from build123d import *

# Parameters (mm, degrees)
SKETCH1_W           = 203.2
SKETCH1_H           = 152.4
BOSS_EXTRUDE1_DEPTH = 12.7
SKETCH2_R           = 2.778125
CUT_EXTRUDE1_DEPTH  = 255.31730181
LPATTERN1_COUNT     = 4
LPATTERN1_PITCH     = 50.8
SKETCH4_R           = 2.778125
SKETCH4_R_2         = 3.175
CUT_EXTRUDE2_DEPTH  = 255.31730181


with BuildPart() as part:
    # Sketch1 → Boss-Extrude1 (new body)
    with BuildSketch(Plane(origin=(0, 0, 0), x_dir=(1, 0, 0), z_dir=(0, 1, 0))):
        with Locations((101.6, 76.2)):
            Rectangle(SKETCH1_W, SKETCH1_H)
    extrude(amount=BOSS_EXTRUDE1_DEPTH)

    # Sketch2 → Cut-Extrude1 (cut, through all)
    with BuildSketch(Plane(origin=(0, 12.7, 0), x_dir=(1, 0, 0), z_dir=(0, 1, 0))):
        with Locations(Location((25.4, 139.7, 0), (0, 0, 270))):
            Circle(SKETCH2_R)
        with Locations(Location((25.4, 12.7, 0), (0, 0, 270))):
            Circle(SKETCH2_R)
    cut_extrude1 = extrude(amount=-CUT_EXTRUDE1_DEPTH, mode=Mode.SUBTRACT)

    # LPattern1: Cut-Extrude1 ×4
    with Locations(*[(i * LPATTERN1_PITCH, 0, 0) for i in range(1, LPATTERN1_COUNT)]):
        add(cut_extrude1, mode=Mode.SUBTRACT)

    # Sketch4 → Cut-Extrude2 (cut, through all)
    with BuildSketch(Plane(origin=(0, 12.7, 0), x_dir=(1, 0, 0), z_dir=(0, 1, 0))):
        with Locations(Location((53.975, 76.2, 0), (0, 0, 270))):
            Circle(SKETCH4_R)
        with Locations(Location((53.34, 107.95, 0), (0, 0, 270))):
            Circle(SKETCH4_R)
        with Locations(Location((101.6, 50.8, 0), (0, 0, 270))):
            Circle(SKETCH4_R_2)
        with Locations(Location((142.875, 107.95, 0), (0, 0, 270))):
            Circle(SKETCH4_R)
        with Locations(Location((136.525, 53.975, 0), (0, 0, 270))):
            Circle(SKETCH4_R)
    extrude(amount=-CUT_EXTRUDE2_DEPTH, mode=Mode.SUBTRACT)


solid = part.part
Can you work these out from the model? Positions are in its coordinate system, mm. Coordinates: 2 decimals unless noted, no trailing zeros. Write each loop counter-clockwise with the first axis right and the second up, starting at its lowest first coordinate (ties: lowest second). Pieces come first, ordered by that corner, then holes. Notation, with made-up numbers: (-26, 68) -> (12, 68) arc R7 ccw to (12, 81) -> close; hole circle Ø3 at (-38.75, 10.25). An arc over 180 degrees is marked (long way). Write each question's results on one line, items separated by ' | '. Start each with the question number.
Q1. We'd pull the mould along Z, two halves only. Please class faces 1 (the face through (73.735, 6.439, -138.418)), 2 (the face through (0, 6, -75)), 3 (the face through (100, 6, -152.4)): +Z half, -Z half, draft (parallel to the pull), parting line (faces both ways), or undercut.
Q2. I'm going to push flat-ended pins straight in: pin 1 (3.5 mm diameter, centred on x = 142.875, z = -107.95, fed in from -Y); pin 2 (7 mm diameter, centred on x = 25.4, z = -139.7, fed in from -Y). Where does each tip first touch, or does it pass through?
Q3. Imagine slicing it at B-B (z = -12.7). Write out the boundary of the cut face in (x, y), then the cut area to 3 significant figures.
Q4. Imagine slicing it at A-A (x = 177.8). Write out the boundary of the cut face in (y, z), then the cut area to 3 significant figures.
Q5. If I drill on probe 1 along X at (y, z) = (1.25, -139.5); probe 2 along Z at (x, y) = (177.8, 9.25); probe 3 along X at (y, z) = (7.25, -107.95), over which ranges is the centre line in solid material (lowest first)?
Taken from the geometry:
1) face 1: undercut | face 2: draft | face 3: -Z half
2) pin 1: passes through | pin 2: stops at y = 0
3) outline: (0, 0) -> (22.62, 0) -> (22.62, 12.7) -> (0, 12.7) -> close; (28.18, 0) -> (73.42, 0) -> (73.42, 12.7) -> (28.18, 12.7) -> close; (78.98, 0) -> (124.22, 0) -> (124.22, 12.7) -> (78.98, 12.7) -> close; (129.78, 0) -> (175.02, 0) -> (175.02, 12.7) -> (129.78, 12.7) -> close; (180.58, 0) -> (203.2, 0) -> (203.2, 12.7) -> (180.58, 12.7) -> close | area: 2,300 mm^2
4) outline: (0, -152.4) -> (12.7, -152.4) -> (12.7, -142.48) -> (0, -142.48) -> close; (0, -136.92) -> (12.7, -136.92) -> (12.7, -15.48) -> (0, -15.48) -> close; (0, -9.92) -> (12.7, -9.92) -> (12.7, 0) -> (0, 0) -> close | area: 1,790 mm^2
5) probe 1: x = 0 to 22.63, 28.17 to 73.43, 78.97 to 124.23, 129.77 to 175.03, 180.57 to 203.2 | probe 2: z = -152.4 to -142.48, -136.92 to -15.48, -9.92 to 0 | probe 3: x = 0 to 50.56, 56.12 to 140.1, 145.65 to 203.2
